```python
from build123d import *

# Parameters (mm, degrees)
SKETCH_2_R               = 15
SKETCH_3_R               = 12.5
CUT_EXTRUDE_1_DEPTH      = 477.393401595
CUT_EXTRUDE_1_DEPTH_BACK = 477.393401595
CUT_EXTRUDE_2_DEPTH      = 477.393401595
CUT_EXTRUDE_2_DEPTH_BACK = 477.393401595
SKETCH_8_R               = 12.88885
CUT_EXTRUDE_1048_DEPTH   = 464.426364673


with BuildPart() as part:
    # Sweep 1: sweep along a path in Sketch 1
    with BuildLine(Plane.XY) as sweep_1_path:
        Line((0, 0), (-163.954760295, -321.779334982))
        ThreePointArc((-163.954760295, -321.779334982), (-189.750317458, -349.684811505), (-226.325216988, -360))
        Line((-226.325216988, -360), (-293.429161818, -360))
    # Sketch 2 → Sweep 1 (sweep)
    with BuildSketch(Plane(origin=(-293.429161818, -360, 0), x_dir=(0, 0, 1), z_dir=(-1, 0, 0))):
        Circle(SKETCH_2_R)
    sweep(path=sweep_1_path.line)

    # Sweep 1 2: sweep along a path in Sketch 1_2
    with BuildLine(Plane.XY) as sweep_1_2_path:
        Line((0, 0), (-163.954760295, -321.779334982))
        ThreePointArc((-163.954760295, -321.779334982), (-189.750317458, -349.684811505), (-226.325216988, -360))
        Line((-226.325216988, -360), (-293.429161818, -360))
    # Sketch 3 → Sweep 1 2 (sweep, cut)
    with BuildSketch(Plane.ZY.offset(293.429161818)):
        with Locations((0, -360)):
            Circle(SKETCH_3_R)
    sweep(path=sweep_1_2_path.line, mode=Mode.SUBTRACT)

    # Sketch 4 → Cut-Extrude 1 (cut, two sides: drawn at the far end of the back side and taken through both)
    with BuildSketch(Plane.XY.offset(-CUT_EXTRUDE_1_DEPTH_BACK)):
        Polygon((-263.429161818, -345), (-293.429161818, -375), (-293.429161818, -345), align=None)
    extrude(amount=CUT_EXTRUDE_1_DEPTH + CUT_EXTRUDE_1_DEPTH_BACK, mode=Mode.SUBTRACT)

    # Sketch 5 → Cut-Extrude 2 (cut, two sides: drawn at the far end of the back side and taken through both)
    with BuildSketch(Plane(origin=(0, 0, 0), x_dir=(0, 0, -1), z_dir=(1, 0, 0)).offset(-CUT_EXTRUDE_2_DEPTH_BACK)):
        with BuildLine():
            Line((-15, 0), (-15, 6.809857496))
            Line((-15, 6.809857496), (15, 6.809857496))
            Line((15, 6.809857496), (15, 0))
            ThreePointArc((15, 0), (0, -15), (-15, 0))
        make_face()
    extrude(amount=CUT_EXTRUDE_2_DEPTH + CUT_EXTRUDE_2_DEPTH_BACK, mode=Mode.SUBTRACT)

    # Sketch 8 → Cut-Extrude 1048 (cut, through all)
    with BuildSketch(Plane(origin=(0, -331.983389073, -120.832071893), x_dir=(1, 0, 0), z_dir=(0, -0.9396926207859081, -0.34202014332566943))):
        with Locations(Location((-243.429161818, 123.127251597, 0), (0, 0, 270))):
            Circle(SKETCH_8_R)
    extrude(amount=-CUT_EXTRUDE_1048_DEPTH, mode=Mode.SUBTRACT)


solid = part.part
```
For this review, take the finished solid that the model builds, in its own axes (mm). A direction names the side the tool comes from. Give positions to 0.01 mm unless a question says otherwise; leave off trailing zeros. One line per item, written item: value. Start each with the question number.
Q1. For L1, parallel to Z at x = -267, y = -360; L2, parallel to Y at x = -275, z = 0; L3, parallel to X at y = -244, z = 6, list the stretches that pass through material, from the lowest coordinate up.
Q2. Add section A-A (z = 0). Count the separate pieces of the cut face and the enclosed holes in it, and give its area (3 significant figures).
Q3. Clearance check with flat-ended pins moving along their axes: pin 1 Ø2 at (y, z) = (-303.5, -11.5) entering from -X; pin 2 Ø6 at (y, z) = (-112.5, 10) entering from -X; pin 3 Ø5 at (x, z) = (-193, 10.5) entering from +Y. State where each tip first meets the part, or that it passes through.
Q4. Draft analysis for pull direction Z (two halves, no side actions). For faces 3 (the face through (-70.078, -169.79, -3.252)), 4 (the face through (3.5, -11.56, 9.56)), 5 (the face through (-275.03, -356.6, -12.29)), state which applies: released by +Z, released by -Z, zero draft, split by the parting line, or undercut.
Q5. Machinability: for faces 1 (the face through (-74.106, -172.32, -2.71)), 2 (the face through (-260.347, -374.643, -3.252)), which of the approach directions +Z, -Z, +X, -X, +Y, -Y give a long, thin tool a straight path to every point of the face, cutting with its end or side? Answer none if there is none.
Reply:
1. L1: -15 to -12.5, 12.5 to 15
1. L2: -375 to -372.5
1. L3: -139.75 to -136.63, -112.02 to -108.89
2. separate pieces: 4
2. enclosed holes: 0
2. area: 2,250 mm²
3. pin 1: x = -166.77
3. pin 2: x = -72.75
3. pin 3: y = -335.92
4. face 3: split by the parting line
4. face 4: undercut
4. face 5: zero draft
5. face 1: none
5. face 2: -X
